from build123d import *

# Parameters (mm, degrees)
F1_DEPTH = 2.5
F2_R     = 1.75
F3_DEPTH = 2.5
F4_R     = 2.35
F4_R_2   = 2
F5_DEPTH = 2.5
F6_W     = 28
F6_H     = 48
F6_R     = 1.5
F7_DEPTH = 2.5


with BuildPart() as f1:
    # F0 (on Top) → F1 (new body)
    with BuildSketch(Plane.XY):
        with BuildLine():
            Line((58, 55), (-58, 55))
            ThreePointArc((-58, 55), (-59.414214, 54.414214), (-60, 53))
            Line((-60, 53), (-60, -53))
            ThreePointArc((-60, -53), (-59.414214, -54.414214), (-58, -55))
            Line((-58, -55), (58, -55))
            ThreePointArc((58, -55), (59.414214, -54.414214), (60, -53))
            Line((60, -53), (60, 53))
            ThreePointArc((60, 53), (59.414214, 54.414214), (58, 55))
        make_face()
    extrude(amount=F1_DEPTH)

    # F2 (on face) → F3 (cut, through all)
    with BuildSketch(Plane.XY.offset(2.5)):
        with Locations((53.25, 27.25)):
            Circle(F2_R)
        with Locations((0, 48.25)):
            Circle(F2_R)
        with Locations((0, -48.25)):
            Circle(F2_R)
        with Locations((53.25, -27.25)):
            Circle(F2_R)
        with Locations((-53.25, -27.25)):
            Circle(F2_R)
    extrude(amount=-F3_DEPTH, mode=Mode.SUBTRACT)

    # F4 (on face) → F5 (cut, through all)
    with BuildSketch(Plane.XY.offset(2.5)):
        with BuildLine():
            Line((-45, -45.5), (-45, -55))
            Line((-45, -55), (-30, -55))
            Line((-30, -55), (-30, -45.5))
            ThreePointArc((-30, -45.5), (-37.5, -38), (-45, -45.5))
        make_face()
        with Locations((-53.265178, 44.226708)):
            Circle(F4_R)
        with Locations((18.234822, 44.226708)):
            Circle(F4_R)
        with Locations((-53.265178, -27.273292)):
            Circle(F4_R)
        with Locations((18.234822, -27.273292)):
            Circle(F4_R)
        with BuildLine():
            ThreePointArc((-18.921428, -6.457228), (-28.121779, -2.129894), (-32.449114, 7.070458))
            Line((-32.449114, 7.070458), (-41.974786, 7.070458))
            ThreePointArc((-41.974786, 7.070458), (-34.839294, -8.847408), (-18.921428, -15.982901))
            Line((-18.921428, -15.982901), (-18.921428, -6.457228))
        make_face()
        with BuildLine():
            ThreePointArc((-18.921428, -19.988577), (-37.667721, -11.675835), (-45.980463, 7.070458))
            Line((-45.980463, 7.070458), (-55.489148, 7.070458))
            ThreePointArc((-55.489148, 7.070458), (-44.385235, -18.39335), (-18.921428, -29.497263))
            Line((-18.921428, -29.497263), (-18.921428, -19.988577))
        make_face()
        with BuildLine():
            ThreePointArc((-19.223845, 46.438274), (-44.425872, 35.306067), (-55.481741, 10.070458))
            Line((-55.481741, 10.070458), (-45.970581, 10.070458))
            ThreePointArc((-45.970581, 10.070458), (-37.664209, 28.632763), (-19.099009, 36.932665))
            Line((-19.099009, 36.932665), (-19.223845, 46.438274))
        make_face()
        with BuildLine():
            Line((-15.921428, -19.978695), (-15.921428, -29.489856))
            ThreePointArc((-15.921428, -29.489856), (9.421141, -18.326925), (20.458793, 7.070458))
            Line((20.458793, 7.070458), (10.950108, 7.070458))
            ThreePointArc((10.950108, 7.070458), (2.70364, -11.609343), (-15.921428, -19.978695))
        make_face()
        with BuildLine():
            ThreePointArc((-16.108928, 23.410645), (-6.97541, 19.149726), (-2.600086, 10.070458))
            Line((-2.600086, 10.070458), (6.93293, 10.070458))
            ThreePointArc((6.93293, 10.070458), (-0.213218, 25.822952), (-15.983928, 32.92881))
            Line((-15.983928, 32.92881), (-16.108928, 23.410645))
        make_face()
        with BuildLine():
            ThreePointArc((-15.931346, 36.932665), (2.633853, 28.632763), (10.940225, 10.070458))
            Line((10.940225, 10.070458), (20.451386, 10.070458))
            ThreePointArc((20.451386, 10.070458), (9.395517, 35.306067), (-15.806511, 46.438274))
            Line((-15.806511, 46.438274), (-15.931346, 36.932665))
        make_face()
        with BuildLine():
            ThreePointArc((-2.581241, 7.070458), (-6.84216, -2.063059), (-15.921428, -6.438384))
            Line((-15.921428, -6.438384), (-15.921428, -15.971399))
            ThreePointArc((-15.921428, -15.971399), (-0.124773, -8.780865), (6.944431, 7.070458))
            Line((6.944431, 7.070458), (-2.581241, 7.070458))
        make_face()
        with BuildLine():
            Line((-18.921428, 23.410645), (-19.046428, 32.92881))
            ThreePointArc((-19.046428, 32.92881), (-34.817137, 25.822952), (-41.963285, 10.070458))
            Line((-41.963285, 10.070458), (-32.430269, 10.070458))
            ThreePointArc((-32.430269, 10.070458), (-28.054945, 19.149726), (-18.921428, 23.410645))
        make_face()
        with Locations((-50, -50)):
            Circle(F4_R_2)
        with Locations((-25, -50)):
            Circle(F4_R_2)
    extrude(amount=-F5_DEPTH, mode=Mode.SUBTRACT)

    # F6 (on face) → F7 (cut, through all)
    with BuildSketch(Plane.XY.offset(2.5)):
        with Locations((36.588879, 0)):
            Rectangle(F6_W, F6_H)
        with Locations((56.588879, 0)):
            Circle(F6_R)
    extrude(amount=-F7_DEPTH, mode=Mode.SUBTRACT)


solid = f1.part
Work out the finished part from the listing and answer in its coordinate system (mm). A direction names the side the tool comes from. Coordinates: 2 decimals unless noted, no trailing zeros. Loops run counter-clockwise (first coordinate to the right, second up) from the corner with the lowest first, then second, coordinate; pieces in that order, holes last. Notation, with made-up numbers: (2.25, 4.25) -> (39.25, 4.25) arc R14 ccw to (39.25, 11.25) -> close; hole circle Ø11 at (-4, 61.25). An arc over 180 degrees is marked (long way). Answer as CSV lines item,"result".
1) For faces 3 (the face through (-60, 1, 1)), 4 (the face through (-30, -50, 1)), 5 (the face through (-44.665, -18.11, 1.268)), determine the directions among +Z, -Z, +X, -X, +Y, -Y from which every point of the face is accessible in a straight line to the end or side of a thin tool.
A:
face 3,"+Z, -Z, -X, +Y, -Y"
face 4,"+Z, -Z, -Y"
face 5,"+Z, -Z"
2) Straight lines are drawn through the part: probe 1 along Y at (x, z) = (53.25, 0.85); probe 2 along Y at (x, z) = (26.5, 1.55); probe 3 along Y at (x, z) = (-14, 0.45). For each, find the intervals that lie inside material, in ascending order.
A:
probe 1,"y = -55 to -29, -25.5 to 25.5, 29 to 55"
probe 2,"y = -55 to -24, 24 to 55"
probe 3,"y = -55 to -29.36, -19.81 to -15.77, -6.11 to 23.06, 32.72 to 36.76, 46.31 to 55"
3) The part is cut by section C-C (x = 26). Give the vertices of the cut face in (y, z).
A:
outline,"(-55, 0) -> (-24, 0) -> (-24, 2.5) -> (-55, 2.5) -> close; (24, 0) -> (55, 0) -> (55, 2.5) -> (24, 2.5) -> close"
4) The part is cut by section B-B (y = 48.25). Give the vertices of the cut face in (x, z), and give its area (3 significant figures).
A:
outline,"(-60, 0) -> (-1.75, 0) -> (-1.75, 2.5) -> (-60, 2.5) -> close; (1.75, 0) -> (60, 0) -> (60, 2.5) -> (1.75, 2.5) -> close"
area,"291 mm²"
5) The part is cut by section D-D (y = 14.5). Give the vertices of the cut face in (x, z), and give its area (3 significant figures).
A:
outline,"(-60, 0) -> (-55.03, 0) -> (-55.03, 2.5) -> (-60, 2.5) -> close; (-45.37, 0) -> (-41.26, 0) -> (-41.26, 2.5) -> (-45.37, 2.5) -> close; (-31.25, 0) -> (-3.78, 0) -> (-3.78, 2.5) -> (-31.25, 2.5) -> close; (6.23, 0) -> (10.34, 0) -> (10.34, 2.5) -> (6.23, 2.5) -> close; (20, 0) -> (22.59, 0) -> (22.59, 2.5) -> (20, 2.5) -> close; (50.59, 0) -> (60, 0) -> (60, 2.5) -> (50.59, 2.5) -> close"
area,"132 mm²"
6) The part is cut by section A-A (x = 53.25). Give the vertices of the cut face in (y, z).
A:
outline,"(-55, 0) -> (-29, 0) -> (-29, 2.5) -> (-55, 2.5) -> close; (-25.5, 0) -> (25.5, 0) -> (25.5, 2.5) -> (-25.5, 2.5) -> close; (29, 0) -> (55, 0) -> (55, 2.5) -> (29, 2.5) -> close"
7) For a pull along Y with two mould halves and no side action, classify faces 1 (the face through (2, 10.07, 1)), 2 (the face through (-1, -11, 2.5)) as released by +Y, released by -Y, zero draft, split by the parting line, or undercut.
A:
face 1,"undercut"
face 2,"zero draft"
8) Flat-ended cylindrical pins translate along their axes: pin 1 (3 mm diameter, centred on x = -19, y = -35.5, fed in from -Z); pin 2 (0.8 mm diameter, centred on x = -38, z = 0.5, fed in from -Y). Find the tip coordinate at first contact, or state that the pin passes through.
A:
pin 1,"stops at z = 0"
pin 2,"stops at y = -38.05"
